CAD build for the part. Positions are in the model's coordinates, mm. A direction names the side the tool comes from. Give positions to 0.01 mm unless a question says otherwise; leave off trailing zeros. Loops run counter-clockwise (first coordinate to the right, second up) from the corner with the lowest first, then second, coordinate; pieces in that order, holes last. Notation, with made-up numbers: (-39, 5.5) - (15, 5.5) arc R20 ccw to (15, 9.5) - close; hole circle Ø4 at (29.5, 69.5). An arc over 180 degrees is marked (long way). Return JSON: item names as keys, results as strings.
from build123d import *

# Parameters (mm, degrees)
SKETCH1_R               = 55
BOSS_EXTRUDE1_DEPTH     = 200
SKETCH2_R               = 45
CUT_EXTRUDE1_DEPTH      = 190
SKETCH3_R               = 17.5
CUT_EXTRUDE2_DEPTH      = 1
CUT_EXTRUDE2_DEPTH_BACK = 201
SKETCH4_R               = 5
CUT_EXTRUDE3_DEPTH      = 2
SKETCH5_R               = 22.5
CUT_EXTRUDE4_DEPTH      = 2
CUT_SWEEP1_PROFILE_R    = 2.5
SKETCH58_R              = 2.5
CUT_EXTRUDE5_DEPTH      = 2


with BuildPart() as part:
    # Sketch1 → Boss-Extrude1 (new body)
    with BuildSketch(Plane(origin=(0, 0, 0), x_dir=(0, 0, -1), z_dir=(1, 0, 0))):
        Circle(SKETCH1_R)
    extrude(amount=BOSS_EXTRUDE1_DEPTH)

    # Sketch2 → Cut-Extrude1 (cut)
    with BuildSketch(Plane(origin=(200, 0, 0), x_dir=(0, 0, -1), z_dir=(1, 0, 0))):
        Circle(SKETCH2_R)
    extrude(amount=-CUT_EXTRUDE1_DEPTH, mode=Mode.SUBTRACT)

    # Sketch3 → Cut-Extrude2 (cut, two sides)
    with BuildSketch(Plane.ZY) as cut_extrude2_sk:
        Circle(SKETCH3_R)
    extrude(amount=CUT_EXTRUDE2_DEPTH, mode=Mode.SUBTRACT)
    extrude(cut_extrude2_sk.sketch, amount=-CUT_EXTRUDE2_DEPTH_BACK, mode=Mode.SUBTRACT)

    # Sketch4 → Cut-Extrude3 (cut)
    with BuildSketch(Plane.ZY):
        with Locations((0, 34)):
            Circle(SKETCH4_R)
        with Locations((0, -34)):
            Circle(SKETCH4_R)
    extrude(amount=-CUT_EXTRUDE3_DEPTH, mode=Mode.SUBTRACT)

    # Sketch5 → Cut-Extrude4 (cut)
    with BuildSketch(Plane.ZY):
        Circle(SKETCH5_R)
    extrude(amount=-CUT_EXTRUDE4_DEPTH, mode=Mode.SUBTRACT)

    # Cut-Sweep1: sweep along a path in Sketch57
    with BuildLine(Plane(origin=(105, 0, 0), x_dir=(0, 0, -1), z_dir=(1, 0, 0))) as cut_sweep1_path:
        CenterArc((0, 0), 55, 0, 360)
    # Cut-Sweep1 profile (on start of the path) → Cut-Sweep1 (sweep, cut)
    with BuildSketch(Plane(origin=(105, 0, -55), x_dir=(0, 0, 1), z_dir=(0, 1, 0))):
        Circle(CUT_SWEEP1_PROFILE_R)
    sweep(path=cut_sweep1_path.line, mode=Mode.SUBTRACT)

    # Sketch58 → Cut-Extrude5 (cut)
    with BuildSketch(Plane.ZY.offset(-2)):
        with Locations((0, 34)):
            Circle(SKETCH58_R)
        with Locations((0, -34)):
            Circle(SKETCH58_R)
    extrude(amount=-CUT_EXTRUDE5_DEPTH, mode=Mode.SUBTRACT)


solid = part.part
1. Cut at A-A, the plane y = 0. Write the cut outline in (x, z).
Values follow:
{"outline": "(0, -55) - (102.5, -55) arc R2.5 cw to (107.5, -55) - (200, -55) - (200, -45) - (10, -45) - (10, -17.5) - (2, -17.5) - (2, -22.5) - (0, -22.5) - close; (0, 22.5) - (2, 22.5) - (2, 17.5) - (10, 17.5) - (10, 45) - (200, 45) - (200, 55) - (107.5, 55) arc R2.5 cw to (102.5, 55) - (0, 55) - close"}
2. Drill centre lines: probe 1 along Y at (x, z) = (0.8, 0); probe 2 along Y at (x, z) = (8, 0); probe 3 along Z at (x, y) = (170, 6). Where is each one in solid material? Low to high.
Values follow:
{"probe 1": "y = -55 to -39, -29 to -22.5, 22.5 to 29, 39 to 55", "probe 2": "y = -55 to -17.5, 17.5 to 55", "probe 3": "z = -54.67 to -44.6, 44.6 to 54.67"}
3. Drop flat-ended pins along their axis: P1, Ø1.5, axis at y = 34.5, z = 0.5, coming from the -X side; P2, Ø16, axis at y = -34, z = 0, coming from the +X side; P3, Ø5, axis at y = -33, z = -2.5, coming from the -X side; P4, Ø9, axis at y = 34, z = 0, coming from the -X side. Give the stop position or say it passes through.
Values follow:
{"P1": "stops at x = 4", "P2": "stops at x = 10", "P3": "stops at x = 0", "P4": "stops at x = 2"}
4. Pull direction Z, two halves, no side cores. Call faces 4 (the face through (153.102, -53.692, 11.923)), 5 (the face through (2, 32, 2)), 6 (the face through (4, 34, 0)), 7 (the face through (0, -24, 1)): +Z half, -Z half, draft (parallel to the pull), parting line (faces both ways), or undercut.
Values follow:
{"face 4": "parting line", "face 5": "undercut", "face 6": "undercut", "face 7": "draft"}
5. Which spindle directions (+Z, -Z, +X, -X, +Y, -Y) get a long thin tool onto all of the face, cutting with end or side? Do faces 1 (the face through (200, -40, 21)), 2 (the face through (10, 1, -19)), 3 (the face through (4, -34, 0)). Say none if no direction does.
Values follow:
{"face 1": "+Z, -Z, +X, +Y, -Y", "face 2": "+X", "face 3": "-X"}
6. Cut at B-B, the plane x = 27. Write the cut outline in (y, z).
Values follow:
{"outline": "circle Ø110 at (0, 0); hole circle Ø90 at (0, 0)"}
